Input: part model. Units: mm. Frame: model coordinates. A direction names the side the tool comes from. Coordinates: 2 decimals unless noted, no trailing zeros. Write each loop counter-clockwise with the first axis right and the second up, starting at its lowest first coordinate (ties: lowest second). Pieces come first, ordered by that corner, then holes. Notation, with made-up numbers: M 1,-4.5 L 54,-4.5 A17 cw 54,25.5 Z; hole C -22.75,34.25 d6. An arc over 180 degrees is marked long. Use CSV: the item, a comma, the result in double quotes.
```python
from build123d import *

# Parameters (mm, degrees)
BOSS_EXTRUDE1_DEPTH = 4
BOSS_EXTRUDE2_DEPTH = 12
BOSS_EXTRUDE3_DEPTH = 4
SKETCH4_R           = 2.65
CUT_EXTRUDE1_DEPTH  = 8
SKETCH5_R           = 2.65
CUT_EXTRUDE2_DEPTH  = 8


with BuildPart() as part:
    # Sketch1 → Boss-Extrude1 (new body)
    with BuildSketch(Plane.XY):
        Polygon((0, 0), (0, 30), (30, 30), (30, 22), (8, 0), align=None)
    extrude(amount=BOSS_EXTRUDE1_DEPTH)

    # Sketch2 → Boss-Extrude2 (add)
    with BuildSketch(Plane.XY.offset(4)):
        Polygon((0, 0), (8, 0), (8, 22), (30, 22), (30, 30), (0, 30), align=None)
    extrude(amount=BOSS_EXTRUDE2_DEPTH)

    # Sketch3 → Boss-Extrude3 (add)
    with BuildSketch(Plane.XY.offset(16)):
        Polygon((0, 30), (0, 0), (8, 0), (30, 22), (30, 30), align=None)
    extrude(amount=BOSS_EXTRUDE3_DEPTH)

    # Sketch4 → Cut-Extrude1 (cut)
    with BuildSketch(Plane(origin=(8, 0, 0), x_dir=(0, 0, -1), z_dir=(1, 0, 0))):
        with Locations((-10, 11)):
            Circle(SKETCH4_R)
    extrude(amount=-CUT_EXTRUDE1_DEPTH, mode=Mode.SUBTRACT)

    # Sketch5 → Cut-Extrude2 (cut)
    with BuildSketch(Plane.XZ.offset(-22)):
        with Locations((23, 10)):
            Circle(SKETCH5_R)
    extrude(amount=-CUT_EXTRUDE2_DEPTH, mode=Mode.SUBTRACT)


solid = part.part
```
1. Section C-C (z = 10). Return loops of the section in (x, y), then the cut area to 3 significant figures.
Resolved:
outline,"M 0,0 L 8,0 L 8,8.35 L 0,8.35 Z; M 0,13.65 L 8,13.65 L 8,22 L 20.35,22 L 20.35,30 L 0,30 Z; M 25.65,22 L 30,22 L 30,30 L 25.65,30 Z"
area,"331 mm^2"
2. Mould query, pull axis Z, two halves, no side actions, for faces 1 (the flat face through (12, 19, 0)), 2 (the flat face through (19, 11, 2)), 3 (the flat face through (14, 16, 4)). Classes: pulls with the +Z half, pulls with the -Z half, needs draft (parallel to the pull), parting line crosses it, or undercut.
Resolved:
face 1,"pulls with the -Z half"
face 2,"needs draft"
face 3,"undercut"
3. Material intervals for line 1 (Z direction, x = 23, y = 25); line 2 (Z direction, x = 21.75, y = 21); line 3 (Y direction, x = 5.75, z = 10), sorted ascending. Write a range as [from, to].
Resolved:
line 1,"z = [0, 7.35], [12.65, 20]"
line 2,"z = [0, 4], [16, 20]"
line 3,"y = [0, 8.35], [13.65, 30]"
4. Section A-A (y = 11). Return loops of the section in (x, z), then the cut area to 3 significant figures.
Resolved:
outline,"M 0,0 L 19,0 L 19,4 L 8,4 L 8,7.35 L 0,7.35 Z; M 0,12.65 L 8,12.65 L 8,16 L 19,16 L 19,20 L 0,20 Z"
area,"206 mm^2"
5. Section B-B (x = 23). Return loops of the section in (y, z), then the cut area to 3 significant figures.
Resolved:
outline,"M 15,0 L 30,0 L 30,7.35 L 22,7.35 L 22,4 L 15,4 Z; M 15,16 L 22,16 L 22,12.65 L 30,12.65 L 30,20 L 15,20 Z"
area,"174 mm^2"
6. Section D-D (x = 9.75). Return loops of the section in (y, z), then the cut area to 3 significant figures.
Resolved:
outline,"M 1.75,0 L 30,0 L 30,20 L 1.75,20 L 1.75,16 L 22,16 L 22,4 L 1.75,4 Z"
area,"322 mm^2"
7. Contact query for flat-ended pins moving along their axis: pin 1 Ø6 at (y, z) = (14, 13.5) entering from +X; pin 2 Ø3 at (y, z) = (11, 10) entering from +X; pin 3 Ø12 at (y, z) = (10, 3.5) entering from +X; pin 4 Ø17.5 at (x, y) = (20, 7) entering from -Z. Output: stop coordinate, or through.
Resolved:
pin 1,"stops at x = 23.66"
pin 2,"passes through"
pin 3,"stops at x = 24"
pin 4,"stops at z = 0"
8. Access query for faces 4 (the flat face through (19, 22, 10)), 5 (the flat face through (19, 11, 18)). Directions: +Z, -Z, +X, -X, +Y, -Y. A direction counts if a zero-diameter tool reaches every point of the face in a straight line with its end or side. Return the directions, or none.
Resolved:
face 4,"+X, -Y"
face 5,"+Z, -Z, +X, -Y"
